```python
from build123d import *

# Parameters (mm, degrees)
SKETCH2_W           = 47
SKETCH2_H           = 42
SKETCH2_R           = 2
SKETCH2_R_2         = 11
BOSS_EXTRUDE1_DEPTH = 3
SKETCH2_3_W         = 47
SKETCH2_3_H         = 4
BOSS_EXTRUDE2_DEPTH = 3
SKETCH3_W           = 47
SKETCH3_H           = 2
BOSS_EXTRUDE3_DEPTH = 50
RIB1_REACH          = 84.353
SKETCH8_WALL_W      = 177.312400038
SKETCH8_WALL_H      = 2
RIB2_REACH          = 84.353
SKETCH10_WALL_W     = 177.312400038
SKETCH10_WALL_H     = 2
CUT_EXTRUDE1_DEPTH  = 50


with BuildPart() as part:
    # Sketch2 → Boss-Extrude1 (new body)
    with BuildSketch(Plane.XY):
        with Locations((23.5, 21)):
            Rectangle(SKETCH2_W, SKETCH2_H)
        with Locations((39, 5.5)):
            Circle(SKETCH2_R, mode=Mode.SUBTRACT)
        with Locations((8, 5.5)):
            Circle(SKETCH2_R, mode=Mode.SUBTRACT)
        with Locations((23.5, 21)):
            Circle(SKETCH2_R_2, mode=Mode.SUBTRACT)
        with Locations((39, 36.5)):
            Circle(SKETCH2_R, mode=Mode.SUBTRACT)
        with Locations((8, 36.5)):
            Circle(SKETCH2_R, mode=Mode.SUBTRACT)
    extrude(amount=-BOSS_EXTRUDE1_DEPTH)

    # Sketch2<3> → Boss-Extrude2 (add)
    with BuildSketch(Plane.XY):
        with Locations((23.5, -2)):
            Rectangle(SKETCH2_3_W, SKETCH2_3_H)
    extrude(amount=-BOSS_EXTRUDE2_DEPTH)

    # Sketch3 → Boss-Extrude3 (add)
    with BuildSketch(Plane(origin=(0, 0, -3), x_dir=(-1, 0, 0), z_dir=(0, 0, -1))):
        with Locations((-23.5, -3)):
            Rectangle(SKETCH3_W, SKETCH3_H)
    extrude(amount=BOSS_EXTRUDE3_DEPTH)

    # Sketch8 wall → Rib1 (add, up to next)
    with BuildSketch(Plane(origin=(0, 1.75, -6.75), x_dir=(0, -0.707106781187, -0.707106781187), z_dir=(0, 0.707106781187, -0.707106781187)), mode=Mode.PRIVATE) as rib1_sk1:
        with Locations((0, -1)):
            Rectangle(SKETCH8_WALL_W, SKETCH8_WALL_H)
    rib1_tool1 = extrude(rib1_sk1.sketch, amount=-RIB1_REACH, mode=Mode.PRIVATE) - part.part
    add(rib1_tool1.solids().sort_by_distance((0, 1.75, -6.75))[0])

    # Sketch10 wall → Rib2 (add, up to next)
    with BuildSketch(Plane(origin=(47, 1.75, -6.75), x_dir=(0, -0.707106781187, -0.707106781187), z_dir=(0, 0.707106781187, -0.707106781187)), mode=Mode.PRIVATE) as rib2_sk1:
        with Locations((0, 1)):
            Rectangle(SKETCH10_WALL_W, SKETCH10_WALL_H)
    rib2_tool1 = extrude(rib2_sk1.sketch, amount=-RIB2_REACH, mode=Mode.PRIVATE) - part.part
    add(rib2_tool1.solids().sort_by_distance((47, 1.75, -6.75))[0])

    # Sketch11 → Cut-Extrude1 (cut)
    with BuildSketch(Plane(origin=(0, -2, 0), x_dir=(1, 0, 0), z_dir=(0, 1, 0))):
        with BuildLine():
            Line((9.5, 49.5), (9.5, 10.5))
            ThreePointArc((9.5, 10.5), (8, 9), (6.5, 10.5))
            Line((6.5, 10.5), (6.5, 49.5))
            ThreePointArc((6.5, 49.5), (8, 51), (9.5, 49.5))
        make_face()
        with BuildLine():
            Line((22, 10.5), (22, 49.5))
            ThreePointArc((22, 49.5), (23.5, 51), (25, 49.5))
            Line((25, 49.5), (25, 10.5))
            ThreePointArc((25, 10.5), (23.5, 9), (22, 10.5))
        make_face()
        with BuildLine():
            Line((40.5, 49.5), (40.5, 10.5))
            ThreePointArc((40.5, 10.5), (39, 9), (37.5, 10.5))
            Line((37.5, 10.5), (37.5, 49.5))
            ThreePointArc((37.5, 49.5), (39, 51), (40.5, 49.5))
        make_face()
    extrude(amount=-CUT_EXTRUDE1_DEPTH, mode=Mode.SUBTRACT)


solid = part.part
```
Build history of the part. All positions in model axes, mm. A direction names the side the tool comes from. Round coordinates to 2 decimals unless told otherwise and drop trailing zeros. Write each loop counter-clockwise with the first axis right and the second up, starting at its lowest first coordinate (ties: lowest second). Pieces come first, ordered by that corner, then holes. Notation, with made-up numbers: (-14, 15) - (25, 15) arc R17 cw to (25, 33) - close; hole circle Ø1 at (-18, 54). An arc over 180 degrees is marked (long way). Answer as CSV lines item,"result".
Q1. Pull direction Y, two halves, no side cores. Call faces 1 (the cylindrical face through (7.566, 34.548, -1.479)), 2 (the flat face through (2, 0, -5)): +Y half, -Y half, draft (parallel to the pull), parting line (faces both ways), or undercut.
Report:
face 1,"undercut"
face 2,"draft"
Q2. Drill centre lines: probe 1 along Y at (x, z) = (8, -1.15); probe 2 along Z at (x, y) = (20.5, -1); probe 3 along Y at (x, z) = (43.5, -40). Where is each one in solid material? Low to high. Write a range as [from, to].
Report:
probe 1,"y = [-4, 3.5], [7.5, 34.5], [38.5, 42]"
probe 2,"z = [-3, 0]"
probe 3,"y = [-4, -2]"
Q3. Cut at C-C (y = 21). Write the cut outline in (x, z).
Report:
outline,"(0, -3) - (12.5, -3) - (12.5, 0) - (0, 0) - close; (34.5, -3) - (47, -3) - (47, 0) - (34.5, 0) - close"
Q4. Cut at A-A (x = 39). Write the cut outline in (y, z).
Report:
outline,"(-4, -53) - (-2, -53) - (-2, -51) - (-4, -51) - close; (-4, -9) - (-2, -9) - (-2, -3) - (3.5, -3) - (3.5, 0) - (-4, 0) - close; (7.5, -3) - (34.5, -3) - (34.5, 0) - (7.5, 0) - close; (38.5, -3) - (42, -3) - (42, 0) - (38.5, 0) - close"
Q5. Drop flat-ended pins along their axis: pin 1 (2 mm diameter, centred on x = 11, z = -46.5, fed in from +Y); pin 2 (22 mm diameter, centred on x = 26.5, y = 30, fed in from -Z). Give the stop position or say it passes through.
Report:
pin 1,"stops at y = -2"
pin 2,"stops at z = -3"
Q6. Cut at B-B (z = -18.5). Write the cut outline in (x, y), and give its area (3 significant figures).
Report:
outline,"(0, -4) - (6.5, -4) - (6.5, -2) - (0, -2) - close; (9.5, -4) - (22, -4) - (22, -2) - (9.5, -2) - close; (25, -4) - (37.5, -4) - (37.5, -2) - (25, -2) - close; (40.5, -4) - (47, -4) - (47, -2) - (40.5, -2) - close"
area,"76.0 mm^2"
Q7. Cut at D-D (x = 23.5). Write the cut outline in (y, z).
Report:
outline,"(-4, -53) - (-2, -53) - (-2, -51) - (-4, -51) - close; (-4, -9) - (-2, -9) - (-2, -3) - (10, -3) - (10, 0) - (-4, 0) - close; (32, -3) - (42, -3) - (42, 0) - (32, 0) - close"
Q8. Tool access for faces 3 (the flat face through (18, 11, -3)), 4 (the flat face through (25, -3, -30)), 5 (the flat face through (23, 9, 0)): list every direction of +Z, -Z, +X, -X, +Y, -Y with a clear straight run to the whole face (end or side of a thin tool).
Report:
face 3,"-Z, +Y"
face 4,"+Y, -Y"
face 5,"+Z, +X, -X, +Y, -Y"
